Could you check a few things on this model? Use its own coordinates, in mm. A direction names the side the tool comes from. Round coordinates to 2 decimals unless told otherwise and drop trailing zeros. Write each loop counter-clockwise with the first axis right and the second up, starting at its lowest first coordinate (ties: lowest second). Pieces come first, ordered by that corner, then holes.
```python
from build123d import *

# Parameters (mm, degrees)
SKETCH1_W                      = 36
SKETCH1_H                      = 38
BOSS_EXTRUDE2_DEPTH            = 53
SKETCH3_W                      = 30
SKETCH3_H                      = 35
CUT_EXTRUDE1_DEPTH             = 51
SKETCH4_W                      = 3
SKETCH4_H                      = 30
BOSS_EXTRUDE3_DEPTH            = 33
SKETCH5_W                      = 53
SKETCH5_H                      = 8
CUT_EXTRUDE2_DEPTH             = 52
SKETCH6_W                      = 53
SKETCH6_H                      = 7
BOSS_EXTRUDE4_DEPTH            = 3
CUT_EXTRUDE4_DEPTH             = 79.797208072
CUT_EXTRUDE4_DEPTH_BACK        = 79.797208072
SKETCH8_W                      = 11.5
SKETCH8_H                      = 3
M2_5_TAPPED_HOLE13_D           = 2.05
M2_5_TAPPED_HOLE13_DEPTH       = 3
M2_5_TAPPED_HOLE13_CSINK_D     = 4
M2_5_TAPPED_HOLE13_CSINK_ANGLE = 179
LPATTERN1_COUNT                = 2
LPATTERN1_PITCH                = 24
LPATTERN1_COUNT_DIR2           = 2
LPATTERN1_PITCH_DIR2           = 12
M2_5_TAPPED_HOLE14_D           = 2.05
M2_5_TAPPED_HOLE14_DEPTH       = 2
M2_5_TAPPED_HOLE14_CSINK_D     = 4
M2_5_TAPPED_HOLE14_CSINK_ANGLE = 179
LPATTERN2_COUNT                = 2
LPATTERN2_PITCH                = 16
LPATTERN2_COUNT_DIR2           = 2
LPATTERN2_PITCH_DIR2           = 12
M2_5_TAPPED_HOLE15_D           = 2.05
M2_5_TAPPED_HOLE15_CSINK_D     = 4
M2_5_TAPPED_HOLE15_CSINK_ANGLE = 179
LPATTERN3_COUNT                = 2
LPATTERN3_PITCH                = 16
M2_5_TAPPED_HOLE16_D           = 2.05
M2_5_TAPPED_HOLE16_CSINK_D     = 4
M2_5_TAPPED_HOLE16_CSINK_ANGLE = 179
LPATTERN4_COUNT                = 2
LPATTERN4_PITCH                = 24
LPATTERN4_COUNT_DIR2           = 2
LPATTERN4_PITCH_DIR2           = 12
SKETCH45_R                     = 1.833333333
CUT_EXTRUDE5_DEPTH             = 74.396185187
LPATTERN5_COUNT                = 2
LPATTERN5_PITCH                = 35
LPATTERN5_COUNT_DIR2           = 2
LPATTERN5_PITCH_DIR2           = 43
CUT_EXTRUDE6_DEPTH             = 75.551995278
CUT_EXTRUDE6_DEPTH_BACK        = 75.551995278
SKETCH46_W                     = 11.5
SKETCH46_H                     = 3.2


with BuildPart() as part:
    # Sketch1 → Boss-Extrude2 (new body)
    with BuildSketch(Plane(origin=(0, 0, 0), x_dir=(0, 0, -1), z_dir=(1, 0, 0))):
        with Locations((18, 19)):
            Rectangle(SKETCH1_W, SKETCH1_H)
    extrude(amount=BOSS_EXTRUDE2_DEPTH)

    # Sketch3 → Cut-Extrude1 (cut)
    with BuildSketch(Plane(origin=(53, 0, 0), x_dir=(0, 0, -1), z_dir=(1, 0, 0))):
        with Locations((18, 17.5)):
            Rectangle(SKETCH3_W, SKETCH3_H)
    extrude(amount=-CUT_EXTRUDE1_DEPTH, mode=Mode.SUBTRACT)

    # Sketch4 → Boss-Extrude3 (add)
    with BuildSketch(Plane.XY):
        with Locations((51.5, 15)):
            Rectangle(SKETCH4_W, SKETCH4_H)
    extrude(amount=-BOSS_EXTRUDE3_DEPTH)

    # Sketch5 → Cut-Extrude2 (cut)
    with BuildSketch(Plane.XY):
        with Locations((26.5, 34)):
            Rectangle(SKETCH5_W, SKETCH5_H)
    extrude(amount=-CUT_EXTRUDE2_DEPTH, mode=Mode.SUBTRACT)

    # Sketch6 → Boss-Extrude4 (add)
    with BuildSketch(Plane(origin=(0, 0, 0), x_dir=(-1, 0, 0), z_dir=(0, -1, 0))):
        with Locations((-26.5, -3.5)):
            Rectangle(SKETCH6_W, SKETCH6_H)
        with Locations((-26.5, 39.5)):
            Rectangle(SKETCH6_W, SKETCH6_H)
    extrude(amount=-BOSS_EXTRUDE4_DEPTH)

    # Sketch8 → Cut-Extrude4 (cut, two sides: drawn at the far end of the back side and taken through both)
    with BuildSketch(Plane(origin=(0, 0, -43), x_dir=(-1, 0, 0), z_dir=(0, 0, -1)).offset(-CUT_EXTRUDE4_DEPTH_BACK)):
        with Locations((-23.75, 1.5)):
            Rectangle(SKETCH8_W, SKETCH8_H)
    extrude(amount=CUT_EXTRUDE4_DEPTH + CUT_EXTRUDE4_DEPTH_BACK, mode=Mode.SUBTRACT)

    # M2.5 Tapped Hole13
    with Locations(Plane.XY):
        with Locations((10, 23)):
            m2_5_tapped_hole13 = CounterSinkHole(M2_5_TAPPED_HOLE13_D / 2, M2_5_TAPPED_HOLE13_CSINK_D / 2, depth=M2_5_TAPPED_HOLE13_DEPTH, counter_sink_angle=M2_5_TAPPED_HOLE13_CSINK_ANGLE)

    # LPattern1: M2.5 Tapped Hole13 2 × 2
    with Locations(*[(i * LPATTERN1_PITCH, -j * LPATTERN1_PITCH_DIR2, 0) for i in range(LPATTERN1_COUNT) for j in range(LPATTERN1_COUNT_DIR2) if (i, j) != (0, 0)]):
        add(m2_5_tapped_hole13, mode=Mode.SUBTRACT)

    # M2.5 Tapped Hole14
    with Locations(Plane.ZY):
        with Locations((-26, 23)):
            m2_5_tapped_hole14 = CounterSinkHole(M2_5_TAPPED_HOLE14_D / 2, M2_5_TAPPED_HOLE14_CSINK_D / 2, depth=M2_5_TAPPED_HOLE14_DEPTH, counter_sink_angle=M2_5_TAPPED_HOLE14_CSINK_ANGLE)

    # LPattern2: M2.5 Tapped Hole14 2 × 2
    with Locations(*[(0, -j * LPATTERN2_PITCH_DIR2, i * LPATTERN2_PITCH) for i in range(LPATTERN2_COUNT) for j in range(LPATTERN2_COUNT_DIR2) if (i, j) != (0, 0)]):
        add(m2_5_tapped_hole14, mode=Mode.SUBTRACT)

    # M2.5 Tapped Hole15 (through all)
    with Locations(Plane(origin=(53, 0, 0), x_dir=(0, 0, -1), z_dir=(1, 0, 0))):
        with Locations((26, 23)):
            m2_5_tapped_hole15 = CounterSinkHole(M2_5_TAPPED_HOLE15_D / 2, M2_5_TAPPED_HOLE15_CSINK_D / 2, counter_sink_angle=M2_5_TAPPED_HOLE15_CSINK_ANGLE)

    # LPattern3: M2.5 Tapped Hole15 ×2
    with Locations(*[(0, 0, i * LPATTERN3_PITCH) for i in range(1, LPATTERN3_COUNT)]):
        add(m2_5_tapped_hole15, mode=Mode.SUBTRACT)

    # M2.5 Tapped Hole16 (through all)
    with Locations(Plane(origin=(0, 0, -36), x_dir=(-1, 0, 0), z_dir=(0, 0, -1))):
        with Locations((-10, 23)):
            m2_5_tapped_hole16 = CounterSinkHole(M2_5_TAPPED_HOLE16_D / 2, M2_5_TAPPED_HOLE16_CSINK_D / 2, counter_sink_angle=M2_5_TAPPED_HOLE16_CSINK_ANGLE)

    # LPattern4: M2.5 Tapped Hole16 2 × 2
    with Locations(*[(i * LPATTERN4_PITCH, -j * LPATTERN4_PITCH_DIR2, 0) for i in range(LPATTERN4_COUNT) for j in range(LPATTERN4_COUNT_DIR2) if (i, j) != (0, 0)]):
        add(m2_5_tapped_hole16, mode=Mode.SUBTRACT)

    # Sketch45 → Cut-Extrude5 (cut, symmetric)
    with BuildSketch(Plane(origin=(0, 3, 0), x_dir=(1, 0, 0), z_dir=(0, 1, 0))):
        with Locations(Location((8, 39.5, 0), (0, 0, 270))):
            Circle(SKETCH45_R)
    cut_extrude5 = extrude(amount=CUT_EXTRUDE5_DEPTH, both=True, mode=Mode.SUBTRACT)

    # LPattern5: Cut-Extrude5 2 × 2
    with Locations(*[(i * LPATTERN5_PITCH, 0, j * LPATTERN5_PITCH_DIR2) for i in range(LPATTERN5_COUNT) for j in range(LPATTERN5_COUNT_DIR2) if (i, j) != (0, 0)]):
        add(cut_extrude5, mode=Mode.SUBTRACT)

    # Sketch46 → Cut-Extrude6 (cut, two sides: drawn at the far end of the back side and taken through both)
    with BuildSketch(Plane(origin=(0, 0, -36), x_dir=(-1, 0, 0), z_dir=(0, 0, -1)).offset(-CUT_EXTRUDE6_DEPTH_BACK)):
        with Locations((-23.75, 4.6)):
            Rectangle(SKETCH46_W, SKETCH46_H)
    extrude(amount=CUT_EXTRUDE6_DEPTH + CUT_EXTRUDE6_DEPTH_BACK, mode=Mode.SUBTRACT)


solid = part.part
```
Q1. Imagine slicing it at D-D, the plane x = 26. Write out the boundary of the cut face in (y, z), then the cut area to 3 significant figures.
Q2. Imagine slicing it at A-A, the plane z = -26. Write out the boundary of the cut face in (x, y) (1 decimal), then the cut area to 3 significant figures.
Q3. Imagine slicing it at B-B, the plane x = 43. Write out the boundary of the cut face in (y, z).
Q4. On a 3-axis mill with a long thin cutter (end or side, diameter ignored), from which of +Z, -Z, +X, -X, +Y, -Y can I reach the whole of each face in a straight line? I mean faces 5 (the cylindrical face through (1.02, 11.69, -9.24)), 6 (the flat face through (26, 15, -33)), 7 (the flat face through (11, 3, -40)). Say none if no direction works.
Q5. We'd pull the mould along Y, two halves only. Please class faces 1 (the cylindrical face through (1.018, 11.045, -24.976)), 2 (the flat face through (41, 3, 2)), 3 (the flat face through (52, 0, -18)), 4 (the cylindrical face through (1.02, 23.69, -25.24)): pulls with the +Y half, pulls with the -Y half, needs draft (parallel to the pull), parting line crosses it, or undercut.
Q6. If I drill on L1, parallel to Y at x = 10, z = -34 (3 decimals); L2, parallel to X at y = 2.1, z = -39.5; L3, parallel to X at y = 11, z = -35.35 (3 decimals), over which ranges is the centre line in solid material (lowest first)?
Q7. Imagine slicing it at C-C, the plane z = -39.5. Write out the boundary of the cut face in (x, y), then the cut area to 4 significant figures.
Q8. I'm going to push flat-ended pins straight in: pin 1 Ø3 at (x, y) = (14, 10.5) entering from -Z; pin 2 Ø2.5 at (x, z) = (26, -1) entering from -Y; pin 3 Ø10 at (x, z) = (7.5, -25) entering from -Y; pin 4 Ø2 at (x, z) = (46.5, -40.5) entering from +Y. Where does each tip first touch, or does it pass through?
Results found:
1. outline: (6.2, -36) - (30, -36) - (30, -33) - (6.2, -33) - close; (6.2, -3) - (30, -3) - (30, 0) - (6.2, 0) - close
1. area: 143 mm2
2. outline: (0, 0) - (2, 0) - (2, 10) - (0, 10) - (0, 9) - close; (0, 12) - (2, 12) - (2, 22) - (0, 22) - (0, 21) - (0, 13) - close; (0, 24) - (2, 24) - (2, 30) - (0, 30) - (0, 25) - close; (50, 0) - (53, 0) - (53, 21) - (53, 22) - (50, 22) - close; (50, 24) - (53, 24) - (53, 25) - (53, 30) - (50, 30) - close
2. area: 136 mm2
3. outline: (0, -43) - (3, -43) - (3, -41.33) - (0, -41.33) - close; (0, -37.67) - (3, -37.67) - (3, -36) - (30, -36) - (30, -33) - (0, -33) - close; (0, -3) - (30, -3) - (30, 0) - (3, 0) - (3, 1.67) - (0, 1.67) - close; (0, 5.33) - (3, 5.33) - (3, 7) - (0, 7) - close
4. face 5: -X
4. face 6: +Y, -Y
4. face 7: -Z, +X, -X, +Y
5. face 1: undercut
5. face 2: pulls with the +Y half
5. face 3: pulls with the -Y half
5. face 4: undercut
6. L1: y = 0 to 9.975, 12.025 to 21.975, 24.025 to 30
6. L2: x = 0 to 6.17, 9.83 to 18, 29.5 to 41.17, 44.83 to 53
6. L3: x = 0 to 8.975, 11.025 to 32.975, 35.025 to 53
7. outline: (0, 0) - (6.17, 0) - (6.17, 3) - (0, 3) - close; (9.83, 0) - (18, 0) - (18, 3) - (9.83, 3) - close; (29.5, 0) - (41.17, 0) - (41.17, 3) - (29.5, 3) - close; (44.83, 0) - (53, 0) - (53, 3) - (44.83, 3) - close
7. area: 102.5 mm2
8. pin 1: stops at z = -36
8. pin 2: stops at y = 6.2
8. pin 3: passes through
8. pin 4: stops at y = 3
